Input: dimensioned drawing with shaded views. Units: mm. Origin: part minimum x, y, z. A direction names the side the tool comes from. Give positions to 0.01 mm unless a question says otherwise; leave off trailing zeros. Loops run counter-clockwise (first coordinate to the right, second up) from the corner with the lowest first, then second, coordinate; pieces in that order, holes last. Notation, with made-up numbers: (-21, 2) -> (20, 2) arc R35 cw to (20, 40) -> close; hole circle Ø5 at (22, 72). An arc over 180 degrees is marked (long way). Answer as a JSON object with one key per item and string values.
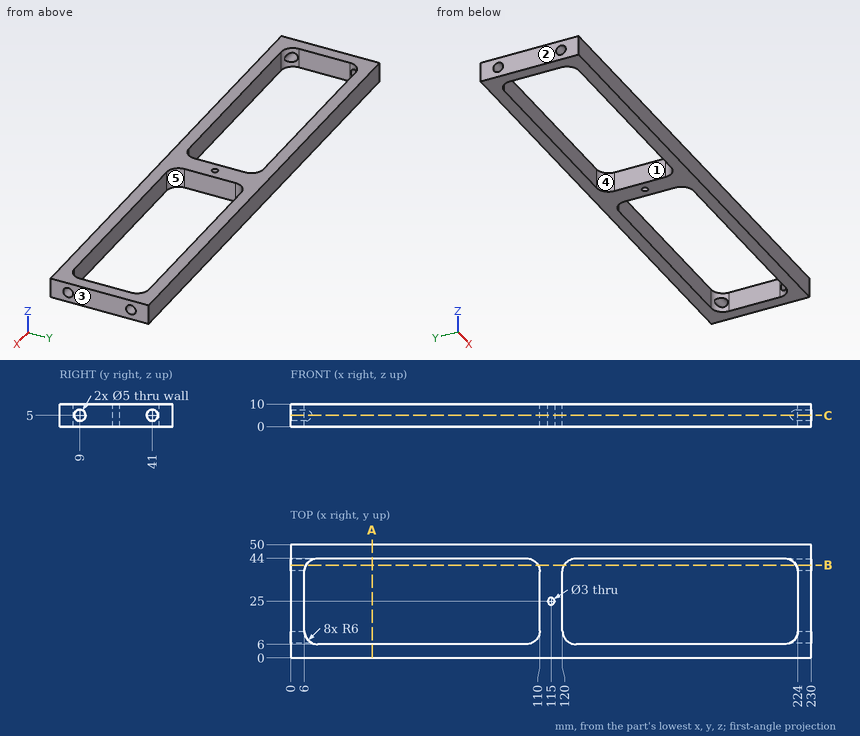
Q1. Draft query along Y for the marked faces 3, 4 and 5. Return one class per face: +Y half, -Y half, draft (parallel to the pull), parting line (faces both ways), or undercut.
Evaluation:
{"face 3": "draft", "face 4": "undercut", "face 5": "undercut"}
Q2. Pin query (flat end, axial travel): pin 1 (4.5 mm diameter, centred on y = 41, z = 5, fed in from -X); pin 2 (5 mm diameter, centred on x = 45.5, z = 3.5, fed in from -Y); pin 3 (4 mm diameter, centred on y = 41, z = 5, fed in from +X). Return the tip coordinate at first contact, or that it passes through.
Evaluation:
{"pin 1": "stops at x = 106.9", "pin 2": "stops at y = 0", "pin 3": "stops at x = 122.68"}
Q3. Ray query, line 1 along X through (y, z) = (28, 8); line 2 along Y through (x, z) = (225, 5); line 3 along Z through (x, y) = (3.25, 41). Return the intervals inside material, ascending.
Evaluation:
{"line 1": "x = 0 to 6, 110 to 120, 224 to 230", "line 2": "y = 0 to 6.5, 11.5 to 38.5, 43.5 to 50", "line 3": "z = 0 to 2.5, 7.5 to 10"}
Q4. Section C-C, the plane z = 5. Give the number of separate pieces and of enclosed holes in the cut face, then the cut area to 3 significant figures.
Evaluation:
{"separate pieces": "3", "enclosed holes": "1", "area": "3,510 mm2"}
Q5. Section A-A, the plane x = 36. Return the cut outline in (y, z), then the cut area to 3 significant figures.
Evaluation:
{"outline": "(0, 0) -> (6, 0) -> (6, 10) -> (0, 10) -> close; (44, 0) -> (50, 0) -> (50, 10) -> (44, 10) -> close", "area": "120 mm2"}
Q6. Section B-B, the plane y = 41. Return the cut outline in (x, z).
Evaluation:
{"outline": "(0, 0) -> (6.8, 0) -> (6.8, 2.5) -> (0, 2.5) -> close; (0, 7.5) -> (6.8, 7.5) -> (6.8, 10) -> (0, 10) -> close; (109.2, 0) -> (120.8, 0) -> (120.8, 10) -> (109.2, 10) -> close; (223.2, 0) -> (230, 0) -> (230, 2.5) -> (223.2, 2.5) -> close; (223.2, 7.5) -> (230, 7.5) -> (230, 10) -> (223.2, 10) -> close"}
Q7. Access query for the marked faces 1 and 2. Directions: +Z, -Z, +X, -X, +Y, -Y. A direction counts if a zero-diameter tool reaches every point of the face in a straight line with its end or side. Return the directions, or none.
Evaluation:
{"face 1": "+Z, -Z", "face 2": "+Z, -Z, -X, +Y, -Y"}
